Solid Edge part; units mm, degrees
sketch "Sketch1" plane through (0, 0, 0) normal (0, 0, 1) x (1, 0, 0)
  line L0 (-15.2, -32.75) -> (15.2, -32.75)
  line L1 (15.2, -32.75) -> (15.2, 32.75)
  line L2 (15.2, 32.75) -> (-15.2, 32.75)
  line L3 (-15.2, 32.75) -> (-15.2, -32.75)
  dimension "D1" = 15.2
  dimension "D2" = 15.2
extrude "Protrusion1" add sketch "Sketch1" along normal blind 1.5
fillet "Verrundung_1" radius 3 4 edges at (15.2, -32.75, 0.75) (-15.2, -32.75, 0.75) (15.2, 32.75, 0.75) (-15.2, 32.75, 0.75)
sketch "Sketch2" plane through (0, 0, 1.5) normal (0, 0, 1) x (0, -1, 0)
  line L0 (-29.9407, 13.1293) -> (-28.0593, 13.1293)
  line L1 (-28.0593, 13.1293) -> (-27.1186, 11.5)
  line L2 (-27.1186, 11.5) -> (-28.0593, 9.8707)
  line L3 (-28.0593, 9.8707) -> (-29.9407, 9.8707)
  line L4 (-30.8814, 11.5) -> (-29.9407, 9.8707)
  line L5 (-30.8814, 11.5) -> (-29.9407, 13.1293)
  line L6 (-29.9407, -9.8707) -> (-28.0593, -9.8707)
  line L7 (-28.0593, -9.8707) -> (-27.1186, -11.5)
  line L8 (-28.0593, -13.1293) -> (-27.1186, -11.5)
  line L9 (-28.0593, -13.1293) -> (-29.9407, -13.1293)
  line L10 (-29.9407, -13.1293) -> (-30.8814, -11.5)
  line L11 (-30.8814, -11.5) -> (-29.9407, -9.8707)
  line L12 (28.0593, 13.1293) -> (29.9407, 13.1293)
  line L13 (29.9407, 13.1293) -> (30.8814, 11.5)
  line L14 (30.8814, 11.5) -> (29.9407, 9.8707)
  line L15 (29.9407, 9.8707) -> (28.0593, 9.8707)
  line L16 (28.0593, 9.8707) -> (27.1186, 11.5)
  line L17 (27.1186, 11.5) -> (28.0593, 13.1293)
  line L18 (28.0593, -9.8707) -> (29.9407, -9.8707)
  line L19 (29.9407, -9.8707) -> (30.8814, -11.5)
  line L20 (30.8814, -11.5) -> (29.9407, -13.1293)
  line L21 (29.9407, -13.1293) -> (28.0593, -13.1293)
  line L22 (28.0593, -13.1293) -> (27.1186, -11.5)
  line L23 (27.1186, -11.5) -> (28.0593, -9.8707)
extrude "Extrusionsausprägung_2" add sketch "Sketch2" along normal blind 9.6 and the other way blind 4
sketch "Sketch3" plane through (0, -32.75, 0.75) normal (0, -1, 0) x (1, 0, 0)
  line L0 (-0.8, 0.75) -> (-0.8, 3.35)
  line L1 (-0.8, 3.35) -> (6, 3.35)
  line L2 (6, 3.35) -> (6, 0.75)
  line L3 (6, 0.75) -> (-0.8, 0.75)
  dimension "D1" = 0.8
  dimension "D2" = 6
extrude "Extrusionsausprägung_3" add sketch "Sketch3" against normal blind 6 and the other way blind 0.5
sketch "Sketch4" plane through (0, 0, 1.5) normal (0, 0, 1) x (0, -1, 0)
  line L0 (-32.75, 6.6) -> (-27.25, 6.6)
  line L1 (-27.25, 6.6) -> (-27.25, -5.8)
  line L2 (-27.25, -5.8) -> (-32.75, -5.8)
  line L3 (-32.75, -5.8) -> (-32.75, 6.6)
  dimension "D1" = 27.25
  dimension "D2" = 27.25
extrude "Extrusionsausprägung_4" add sketch "Sketch4" along normal blind 6
sketch "Sketch5" plane through (0, 32.75, 3.75) normal (0, 1, 0) x (-1, 0, 0)
  line L0 (-3.5, 2.95) -> (-0.6, 2.95)
  line L1 (-0.6, 2.95) -> (-0.6, 0.55)
  line L2 (-0.6, 0.55) -> (-3.5, 0.55)
  line L3 (-3.5, 0.55) -> (-3.5, 2.95)
  dimension "D1" = 3.5
  dimension "D2" = 0.6
extrude "Extrusionsausprägung_5" add sketch "Sketch5" along normal blind 2.5
sketch "Sketch6" plane through (11.5, 29, 11.1) normal (0, 0, 1) x (0, -1, 0)
  circle A0 centre (0, 0) radius 1
  circle A1 centre (0, -23) radius 1
  circle A2 centre (58, -23) radius 1
  circle A3 centre (58, 0) radius 1
extrude "Cutout1" cut sketch "Sketch6" against normal through all
sketch "Sketch7" plane through (0, 0, 0) normal (0, 0, -1) x (0, -1, 0)
  line L0 (-30.25, 8.2) -> (-28.75, 8.2)
  line L1 (-28.75, 8.2) -> (-28.75, -8.3)
  line L2 (-28.75, -8.3) -> (-30.25, -8.3)
  line L3 (-30.25, -8.3) -> (-30.25, 8.2)
  dimension "D1" = 30.25
  dimension "D2" = 28.75
extrude "Extrusionsausprägung_6" add sketch "Sketch7" along normal blind 1.2
sketch "Sketch8" plane through (0, 0, 0) normal (0, 0, -1) x (0, -1, 0)
  line L0 (3.75, 15.2) -> (3.75, -15.2)
  line L1 (3.75, -15.2) -> (26.638, -15.2)
  line L2 (26.638, -15.2) -> (26.638, 7.3196)
  line L3 (26.638, 7.3196) -> (29.2171, 7.3196)
  line L4 (29.2171, 7.3196) -> (29.2171, 9.2846)
  line L5 (29.2171, 9.2846) -> (26.638, 9.2846)
  line L6 (26.638, 9.2846) -> (26.638, 15.2)
  line L7 (26.638, 15.2) -> (3.75, 15.2)
extrude "Extrusionsausprägung_7" add sketch "Sketch8" along normal blind 2
The model under review builds one solid part; all positions refer to its coordinate system, in mm. A direction names the side the tool comes from. Round coordinates to 2 decimals unless told otherwise and drop trailing zeros. Order: outer loops, then holes, each group sorted by start corner. A loop starts at its lowest first (then second) coordinate and runs counter-clockwise, first axis right, second up. Notation, with made-up numbers: (36, -40) -> (80, -40) arc R28 ccw to (80, -7) -> close; hole circle Ø6 at (55.25, 0.5). An arc over 180 degrees is marked (long way). Use a Markdown table: item, result.
Q1. Clearance check with flat-ended pins moving along their axes: P1, Ø0.9, axis at y = 29.5, z = -1, coming from the +X side; P2, Ø8, axis at x = 10, z = -0.5, coming from the +Y side; P3, Ø1.6, axis at x = -13, z = -0.5, coming from the -Y side. State where each tip first meets the part, or that it passes through.
Values:
| item | result |
|---|---|
| P1 | stops at x = 13.13 |
| P2 | stops at y = 32.75 |
| P3 | stops at y = -32.74 |
Q2. For line 1 (X direction, y = -29, z = 7); line 2 (X direction, y = 29, z = 2); line 3 (X direction, y = -29, z = 3.25), list the stretches that pass through material, from the lowest coordinate up.
Values:
| item | result |
|---|---|
| line 1 | x = -13.13 to -12.5, -10.5 to -9.87, 9.87 to 10.5, 12.5 to 13.13 |
| line 2 | x = -13.13 to -12.5, -10.5 to -9.87, -5.8 to 6.6, 9.87 to 10.5, 12.5 to 13.13 |
| line 3 | x = -13.13 to -12.5, -10.5 to -9.87, -0.8 to 6, 9.87 to 10.5, 12.5 to 13.13 |
Q3. Mouldability with a two-part tool opening along X and no side actions: class faces 6 (the flat face through (-13.129, 29, 6)), 7 (the flat face through (-11.5, 27.8, -2.5)), 8 (the flat face through (12.3, 30.42, -1.27)), 9 (the flat face through (-10.7, 30.42, 6.23)) as +X half, -X half, draft (parallel to the pull), parting line (faces both ways), or undercut.
Values:
| item | result |
|---|---|
| face 6 | -X half |
| face 7 | draft |
| face 8 | +X half |
| face 9 | undercut |
Q4. We need section D-D on y = -11. Write out the cut boundary in (x, z).
Values:
| item | result |
|---|---|
| outline | (-15.2, -2) -> (15.2, -2) -> (15.2, 1.5) -> (-15.2, 1.5) -> close |
Q5. We need section A-A on z = 8.5. Write out the cut boundary in (x, y), then the cut area to 3 significant figures.
Values:
| item | result |
|---|---|
| outline | (-13.13, -29.94) -> (-11.5, -30.88) -> (-9.87, -29.94) -> (-9.87, -28.06) -> (-11.5, -27.12) -> (-13.13, -28.06) -> close; (-13.13, 28.06) -> (-11.5, 27.12) -> (-9.87, 28.06) -> (-9.87, 29.94) -> (-11.5, 30.88) -> (-13.13, 29.94) -> close; (9.87, -29.94) -> (11.5, -30.88) -> (13.13, -29.94) -> (13.13, -28.06) -> (11.5, -27.12) -> (9.87, -28.06) -> close; (9.87, 28.06) -> (11.5, 27.12) -> (13.13, 28.06) -> (13.13, 29.94) -> (11.5, 30.88) -> (9.87, 29.94) -> close; hole circle Ø2 at (-11.5, -29); hole circle Ø2 at (-11.5, 29); hole circle Ø2 at (11.5, -29); hole circle Ø2 at (11.5, 29) |
| area | 24.2 mm^2 |
Q6. We need section B-B on z = 2.25. State how many separate pieces and enclosed holes the cut face has, then the cut area to 3 significant figures.
Values:
| item | result |
|---|---|
| separate pieces | 6 |
| enclosed holes | 4 |
| area | 137 mm^2 |
Q7. We need section C-C on x = -4. Write out the cut boundary in (y, z), then the cut area to 3 significant figures.
Values:
| item | result |
|---|---|
| outline | (-32.75, 0) -> (-26.64, 0) -> (-26.64, -2) -> (-3.75, -2) -> (-3.75, 0) -> (28.75, 0) -> (28.75, -1.2) -> (30.25, -1.2) -> (30.25, 0) -> (32.75, 0) -> (32.75, 7.5) -> (27.25, 7.5) -> (27.25, 1.5) -> (-32.75, 1.5) -> close |
| area | 179 mm^2 |
Q8. Tool access review of faces 1 (the flat face through (10.7, -30.42, 6.23)), 2 (the flat face through (10.7, 27.58, 6.23)), 3 (the flat face through (-9.285, -28, -1)), 4 (the flat face through (2, 34, 4.3)), 5 (the flat face through (10.7, 27.58, -1.27)): name each direction out of +Z, -Z, +X, -X, +Y, -Y from which nothing blocks a thin tool from reaching the whole face with its end or side.
Values:
| item | result |
|---|---|
| face 1 | +Z, -Y |
| face 2 | +Z |
| face 3 | -Z, -Y |
| face 4 | -Z, +X, -X, +Y |
| face 5 | -Z |
